Design review of the part built by this model. Coordinates are the model's own, in mm. A direction names the side the tool comes from. Give positions to 0.01 mm unless a question says otherwise; leave off trailing zeros. Loops run counter-clockwise (first coordinate to the right, second up) from the corner with the lowest first, then second, coordinate; pieces in that order, holes last. Notation, with made-up numbers: M 56,9.25 L 82,9.25 A16 cw 82,19.25 Z; hole C 21.5,50.5 d8. An arc over 180 degrees is marked long. Use CSV: the item, a comma, the result in double quotes.
from build123d import *

# Parameters (mm, degrees)
F0_R     = 9.525
F1_DEPTH = 41.275
F2_R     = 19.431
F3_DEPTH = 9.525
F4_W     = 127
F4_H     = 127
F5_DEPTH = 87.63
F6_SIZE  = 19.05
F7_R     = 42.926
F8_DEPTH = 199.644


with BuildPart() as f1:
    # F0 (on Front) → F1 (new body)
    with BuildSketch(Plane.XZ):
        Circle(F0_R)
    extrude(amount=F1_DEPTH)

    # F2 (on face) → F3 (join)
    with BuildSketch(Plane(origin=(0, 0, 0), x_dir=(-1, 0, 0), z_dir=(0, 1, 0))):
        Circle(F2_R)
    extrude(amount=F3_DEPTH)

    # F4 (on face) → F5 (join)
    with BuildSketch(Plane(origin=(0, 9.525, 0), x_dir=(-1, 0, 0), z_dir=(0, 1, 0))):
        with Locations((0, -22.86)):
            Rectangle(F4_W, F4_H)
    extrude(amount=F5_DEPTH)

    # F6
    f6_edges = [f1.edges().sort_by_distance(p)[0] for p in [
        (63.5, 53.34, 40.64),
        (-63.5, 53.34, 40.64),
        (63.5, 53.34, -86.36),
        (-63.5, 53.34, -86.36),
    ]]
    chamfer(f6_edges, length=F6_SIZE)

    # F7 (on face) → F8 (join)
    with BuildSketch(Plane(origin=(0, 97.155, 0), x_dir=(-1, 0, 0), z_dir=(0, 1, 0))):
        with Locations((0, -22.86)):
            Circle(F7_R)
    extrude(amount=F8_DEPTH)


solid = f1.part
(1) Wall thickness on line 1 along Y through (x, z) = (30, -2) (3 decimals); line 2 along Y through (x, z) = (-54.5, 21) (3 decimals); line 3 along X through (y, z) = (232.5, -21.5): over which ranges is each line inside the solid? List them lowest first. Write a range as [from, to].
A:
line 1,"[9.525, 296.799]"
line 2,"[9.525, 97.155]"
line 3,"[-42.9, 42.9]"
(2) We need section A-A on z = -22.86. State the section outline as (x, y) points (3 decimals), then the cut area to 3 significant figures.
A:
outline,"M -63.5,9.525 L 63.5,9.525 L 63.5,97.155 L 42.926,97.155 L 42.926,296.799 L -42.926,296.799 L -42.926,97.155 L -63.5,97.155 Z"
area,"28,300 mm²"
(3) Clearance check with flat-ended pins moving along their axes: P1, Ø2, axis at x = -29.5, y = 257.5, coming from the +Z side; P2, Ø1, axis at y = 251.5, z = -45, coming from the +X side; P3, Ø3, axis at y = 125, z = -61, coming from the -X side. State where each tip first meets the part, or that it passes through.
A:
P1,"z = 9.24"
P2,"x = 37.07"
P3,"x = -22.36"
(4) We need section C-C on y = 249. State the section outline as (x, z) points.
A:
outline,"C 0,-22.86 d85.85"
(5) Machinability: for faces 1 (the flat face through (-54.11, 52.73, 30.98)), 2 (the cylindrical face through (-23.077, 195.579, 13.335)), 3 (the cylindrical face through (-7.559, -20.349, -5.796)), which of the approach directions +Z, -Z, +X, -X, +Y, -Y give a long, thin tool a straight path to every point of the face, cutting with its end or side? Answer none if there is none.
A:
face 1,"+Z, -X, +Y, -Y"
face 2,"+Y"
face 3,"-Y"
(6) We need section D-D on z = 3.5. State the section outline as (x, y) points (3 decimals).
A:
outline,"M -63.5,9.525 L -19.113,9.525 L -19.113,0 L -8.859,0 L -8.859,-41.275 L 8.859,-41.275 L 8.859,0 L 19.113,0 L 19.113,9.525 L 63.5,9.525 L 63.5,97.155 L 33.879,97.155 L 33.879,296.799 L -33.879,296.799 L -33.879,97.155 L -63.5,97.155 Z"
(7) We need section B-B on x = 0. State the section outline as (y, z) points (3 decimals), then the cut area to 3 significant figures.
A:
outline,"M -41.275,-9.525 L 0,-9.525 L 0,-19.431 L 9.525,-19.431 L 9.525,-86.36 L 97.155,-86.36 L 97.155,-65.786 L 296.799,-65.786 L 296.799,20.066 L 97.155,20.066 L 97.155,40.64 L 9.525,40.64 L 9.525,19.431 L 0,19.431 L 0,9.525 L -41.275,9.525 Z"
area,"29,400 mm²"
